Verification items for this drawing (mm, ordinates from the low corner). A direction names the side the tool comes from. Give positions to 0.01 mm unless a question says otherwise; leave off trailing zeros. Loops run counter-clockwise (first coordinate to the right, second up) from the corner with the lowest first, then second, coordinate; pieces in that order, holes last. Notation, with made-up numbers: M -22,55 L 26,55 A33 cw 26,91 Z; hole C -7,19.25 d4. An arc over 180 degrees is marked long. Use one line per item in the form item = value.
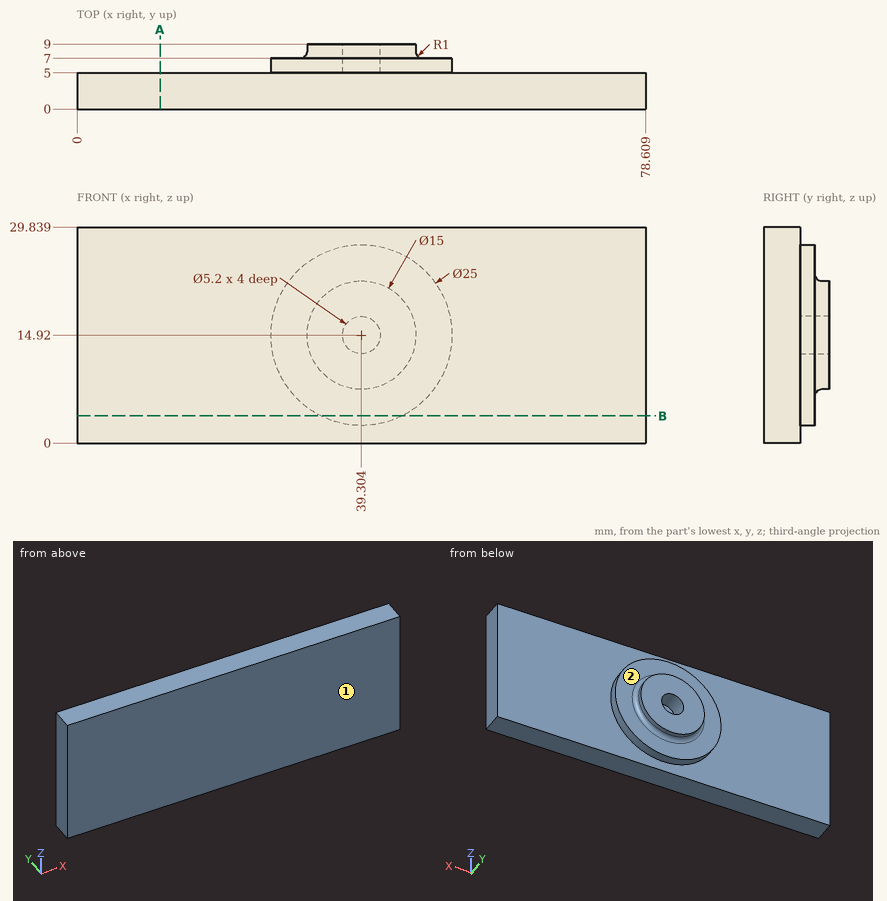
1) Set-up check for the marked faces 1 and 2: record each of +Z, -Z, +X, -X, +Y, -Y from which the full face is reachable in a straight line by a thin tool's end or side.
Evaluation:
face_1 = +Z, -Z, +X, -X, -Y
face_2 = +Y
2) Scan lines: line 1 (Y direction, x = 68, z = 24.75); line 2 (Y direction, x = 28.5, z = 20.75); line 3 (X direction, y = 8.25, z = 16) (1 decimal). Record each from-to range of solid material in increasing order.
Evaluation:
line_1 = 0 to 5
line_2 = 0 to 7
line_3 = 31.9 to 36.9, 41.7 to 46.7
3) Depth check by flat-ended pin: pin 1 Ø8 at (x, z) = (29.5, 3.5) entering from +Y; pin 2 Ø1.5 at (y, z) = (7.5, 19) entering from -X; pin 3 Ø2.5 at (x, z) = (38.5, 14.5) entering from +Y; pin 4 Ø6 at (x, z) = (49.5, 8) entering from -Y. Enter the tip coordinate at first touch or a pass-through.
Evaluation:
pin_1 = 7
pin_2 = 27.31
pin_3 = 5
pin_4 = 0
4) Section check B-B (z = 3.75). Record the cut outline in (x, y) (1 decimal).
Evaluation:
outline = M 0,0 L 78.6,0 L 78.6,5 L 44.9,5 L 44.9,7 L 33.7,7 L 33.7,5 L 0,5 Z
5) Section check A-A (x = 11.5). Record the cut outline in (y, z), then the cut area to 3 significant figures.
Evaluation:
outline = M 0,0 L 5,0 L 5,29.84 L 0,29.84 Z
area = 149 mm^2
